Input: part model. Units: mm. Frame: model coordinates. Round coordinates to 2 decimals unless told otherwise and drop trailing zeros. Order: outer loops, then holes, each group sorted by start corner. A loop starts at its lowest first (then second) coordinate and runs counter-clockwise, first axis right, second up. Notation, with made-up numbers: (80.25, 17) -> (108.25, 17) arc R19 cw to (108.25, 26) -> close; hole circle Ø10 at (-35, 13.5). An arc over 180 degrees is marked (long way). Use a Markdown table: item, result.
from build123d import *

# Parameters (mm, degrees)
F0_W     = 20.32
F0_H     = 10.16
F1_DEPTH = 6.88
F2_R     = 0.25
F3_DEPTH = 3.05


with BuildPart() as f1:
    # F0 (on Top) → F1 (new body)
    with BuildSketch(Plane.XY):
        Rectangle(F0_W, F0_H)
    extrude(amount=F1_DEPTH)

    # F2 (on face) → F3 (join)
    with BuildSketch(Plane(origin=(0, 0, 0), x_dir=(1, 0, 0), z_dir=(0, 0, -1))):
        with BuildLine():
            ThreePointArc((-7.62, 2.29), (-7.443223, 2.363223), (-7.37, 2.54))
            ThreePointArc((-7.37, 2.54), (-7.796777, 2.716777), (-7.62, 2.29))
        make_face()
        with BuildLine():
            ThreePointArc((-7.37, -2.54), (-7.443223, -2.363223), (-7.62, -2.29))
            ThreePointArc((-7.62, -2.29), (-7.796777, -2.716777), (-7.37, -2.54))
        make_face()
        with Locations((-5.08, 2.54)):
            Circle(F2_R)
        with BuildLine():
            ThreePointArc((7.62, 2.29), (7.796777, 2.363223), (7.87, 2.54))
            ThreePointArc((7.87, 2.54), (7.443223, 2.716777), (7.62, 2.29))
        make_face()
        with BuildLine():
            ThreePointArc((7.87, -2.54), (7.796777, -2.363223), (7.62, -2.29))
            ThreePointArc((7.62, -2.29), (7.443223, -2.716777), (7.87, -2.54))
        make_face()
    extrude(amount=F3_DEPTH)


solid = f1.part
1) Cut plane B-B on y = -0.25. Return loops of the section in (x, z).
Answer key:
| item | result |
|---|---|
| outline | (-10.16, 0) -> (10.16, 0) -> (10.16, 6.88) -> (-10.16, 6.88) -> close |
2) Ray query, probe 1 along Z at (x, y) = (4, -1.5). Return the intervals inside material, ascending.
Answer key:
| item | result |
|---|---|
| probe 1 | z = 0 to 6.88 |
3) Contact query for a flat-ended pin moving along its axis: P1, Ø4, axis at x = 5.5, y = 1, coming from the -Z side. Output: stop coordinate, or through.
Answer key:
| item | result |
|---|---|
| P1 | stops at z = 0 |
4) Cut plane A-A on x = -5.08. Return loops of the section in (y, z), and give its area (3 significant figures).
Answer key:
| item | result |
|---|---|
| outline | (-5.08, 0) -> (-2.79, 0) -> (-2.79, -3.05) -> (-2.29, -3.05) -> (-2.29, 0) -> (5.08, 0) -> (5.08, 6.88) -> (-5.08, 6.88) -> close |
| area | 71.4 mm^2 |
5) Cut plane C-C on x = -1.25. Return loops of the section in (y, z), and give its area (3 significant figures).
Answer key:
| item | result |
|---|---|
| outline | (-5.08, 0) -> (5.08, 0) -> (5.08, 6.88) -> (-5.08, 6.88) -> close |
| area | 69.9 mm^2 |
